Design review of the part built by this model. Coordinates are the model's own, in mm. Face numbers are marked on the shaded views. A direction names the side the tool comes from. Coordinates: 2 decimals unless noted, no trailing zeros. Write each loop counter-clockwise with the first axis right and the second up, starting at its lowest first coordinate (ties: lowest second). Pieces come first, ordered by that corner, then holes.
Q1. Take a section at A-A, the plane x = 81. Write out the cut boundary in (y, z) (3 decimals).
Q2. The part is to be moulded in two halves that separate along Z. For the marked faces 1, 2 and 3, say which applies: released by +Z, released by -Z, zero draft, split by the parting line, or undercut.
Q3. Take a section at C-C, the plane x = 31.75. Write out the cut boundary in (y, z) (3 decimals), plus the area to 3 significant figures.
Q4. For pin 1 Ø5 at (x, y) = (34.5, -14) entering from -Z; pin 2 Ø14 at (x, z) = (56.5, -27) entering from +Y (3 decimals); pin 3 Ø17 at (x, z) = (95.25, 6.6) entering from +Y; pin 4 Ø6.5 at (x, z) = (40.5, -24.5) entering from -Y (3 decimals), all flat-tipped, find the tip position at first contact; note any pin that passes through.
Q5. For the marked faces 4 and 5, list the 3-axis set-ups (+Z, -Z, +X, -X, +Y, -Y) from which the entire face can be reached by the end or side of a thin tool; tool diameter is ignored.
Q6. Take a section at D-D, the plane y = 0. Write out the cut boundary in (x, z) (3 decimals), plus the area to 3 significant figures.
Q7. Take a section at B-B, the plane y = -5.5. Write out the cut boundary in (x, z) (3 decimals), plus the area to 3 significant figures.
Q8. For L1, parallel to X at y = -13, z = 6.5; L2, parallel to Z at x = 95.25, y = 7; L3, parallel to Z at x = 31, y = 11, list the stretches that pass through material, from the lowest coordinate up.
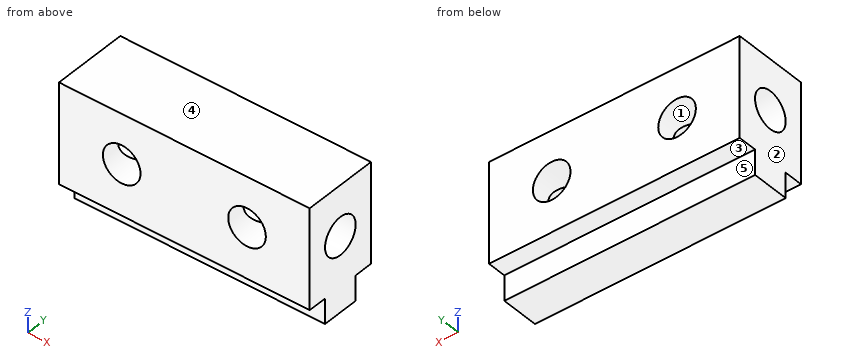
from build123d import *

# Parameters (mm, degrees)
F0_R          = 9.525
F1_DEPTH      = 127
F2_R          = 9.525
F3_DEPTH      = 46.228
F3_DEPTH_BACK = 48.514


with BuildPart() as f1:
    # F0 (on Right) → F1 (new body)
    with BuildSketch(Plane.YZ):
        Polygon((19.05, -19.05), (19.05, 31.75), (-19.05, 31.75), (-19.05, -19.05), (-9.525, -19.05), (-9.525, -31.75), (9.525, -31.75), (9.525, -19.05), align=None)
        with Locations((0, 6.35)):
            Circle(F0_R, mode=Mode.SUBTRACT)
    extrude(amount=F1_DEPTH)

    # F2 (on Front) → F3 (cut, two sides)
    with BuildSketch(Plane.XZ) as f3_sk:
        with Locations((31.75, 6.600567)):
            Circle(F2_R)
        with Locations((95.25, 6.600567)):
            Circle(F2_R)
    extrude(amount=F3_DEPTH, mode=Mode.SUBTRACT)
    extrude(f3_sk.sketch, amount=-F3_DEPTH_BACK, mode=Mode.SUBTRACT)


solid = f1.part
Responses:
1. outline: (-19.05, -19.05) - (-9.525, -19.05) - (-9.525, -31.75) - (9.525, -31.75) - (9.525, -19.05) - (19.05, -19.05) - (19.05, 31.75) - (-19.05, 31.75) - close; hole circle Ø19.05 at (0, 6.35)
2. face 1: undercut
2. face 2: zero draft
2. face 3: released by -Z
3. outline: (-19.05, -19.05) - (-9.525, -19.05) - (-9.525, -31.75) - (9.525, -31.75) - (9.525, -19.05) - (19.05, -19.05) - (19.05, -2.924) - (2.17, -2.924) arc R9.525 cw to (-2.17, -2.924) - (-19.05, -2.924) - close; (-19.05, 16.126) - (19.05, 16.126) - (19.05, 31.75) - (-19.05, 31.75) - close
3. area: 1,450 mm2
4. pin 1: stops at z = -19.05
4. pin 2: stops at y = 9.525
4. pin 3: passes through
4. pin 4: stops at y = -9.525
5. face 4: +Z, +X, -X, +Y, -Y
5. face 5: -Z, +X, -X, +Y
6. outline: (0, -31.75) - (127, -31.75) - (127, -3.175) - (0, -3.175) - close; (0, 15.875) - (29.58, 15.875) arc R9.525 cw to (33.92, 15.875) - (93.08, 15.875) arc R9.525 cw to (97.42, 15.875) - (127, 15.875) - (127, 31.75) - (0, 31.75) - close
6. area: 5,640 mm2
7. outline: (0, -31.75) - (127, -31.75) - (127, -1.427) - (100.377, -1.427) arc R9.525 cw to (90.123, -1.427) - (36.877, -1.427) arc R9.525 cw to (26.623, -1.427) - (0, -1.427) - close; (0, 14.127) - (25.912, 14.127) arc R9.525 cw to (37.588, 14.127) - (89.412, 14.127) arc R9.525 cw to (101.088, 14.127) - (127, 14.127) - (127, 31.75) - (0, 31.75) - close
7. area: 6,040 mm2
8. L1: x = 0 to 22.23, 41.27 to 85.73, 104.77 to 127
8. L2: z = -31.75 to -2.92, 16.13 to 31.75
8. L3: z = -19.05 to -2.89, 16.1 to 31.75
